```python
from build123d import *

# Parameters (mm, degrees)
BOSS_EXTRUDE1_DEPTH            = 20.32
SKETCH2_R                      = 3.175
BOSS_EXTRUDE2_DEPTH            = 69.85
F_3_5_3_5_DIAMETER_HOLE1_D     = 3.5
F_3_5_3_5_DIAMETER_HOLE1_DEPTH = 25.4
F_3_5_3_5_DIAMETER_HOLE1_TIP   = 1.051506083
F_1_16_0_0625_DIAMETER_HOLE1_D = 1.5875


with BuildPart() as part:
    # Sketch1 → Boss-Extrude1 (new body)
    with BuildSketch(Plane.XY):
        Polygon((0, 7.332348419), (-6.35, 3.666174209), (-6.35, -3.666174209), (0, -7.332348419), (6.35, -3.666174209), (6.35, 3.666174209), align=None)
    extrude(amount=BOSS_EXTRUDE1_DEPTH)

    # Sketch2 → Boss-Extrude2 (add)
    with BuildSketch(Plane.XY.offset(20.32)):
        Circle(SKETCH2_R)
    extrude(amount=BOSS_EXTRUDE2_DEPTH)

    # Ø3.5 (3.5) Diameter Hole1
    with Locations(Plane.XY.offset(90.17)):
        with Locations((0, 0)):
            Hole(F_3_5_3_5_DIAMETER_HOLE1_D / 2, depth=F_3_5_3_5_DIAMETER_HOLE1_DEPTH)
            with Locations((0, 0, -(F_3_5_3_5_DIAMETER_HOLE1_DEPTH + F_3_5_3_5_DIAMETER_HOLE1_TIP / 2))):  # 118° drill point
                Cone(0, F_3_5_3_5_DIAMETER_HOLE1_D / 2, F_3_5_3_5_DIAMETER_HOLE1_TIP, mode=Mode.SUBTRACT)

    # 1/16 (0.0625) Diameter Hole1 (through all)
    with Locations(Plane(origin=(0, 7.62, 0), x_dir=(1, 0, 0), z_dir=(0, 1, 0))):
        with Locations((0, -83.82)):
            Hole(F_1_16_0_0625_DIAMETER_HOLE1_D / 2)


solid = part.part
```
The listing builds one solid part. Answer for the finished solid, in the listing's coordinates (mm). A direction names the side the tool comes from. Give positions to 0.01 mm unless a question says otherwise; leave off trailing zeros. Write each loop counter-clockwise with the first axis right and the second up, starting at its lowest first coordinate (ties: lowest second). Pieces come first, ordered by that corner, then holes. Notation, with made-up numbers: (17, 38.5) -> (45, 38.5) arc R21 ccw to (45, 64.5) -> close; hole circle Ø1 at (-27, 18). An arc over 180 degrees is marked (long way). Write item = value, one per line. Start each with the question number.
1) Straight lines are drawn through the part: line 1 along Y through (x, z) = (0, 68.5) (3 decimals); line 2 along Z through (x, y) = (0, -2.4); line 3 along X through (y, z) = (2.3, 83.82). For each, find the intervals that lie inside material, in ascending order.
2) Which of the six approach directions +Z, -Z, +X, -X, +Y, -Y give full straight-line access (tool end or side, diameter ignored) to faces 4 (the face through (-1.617, -0.67, 77.292)), 5 (the face through (3.219, 5.474, 10.018))?
3) The part is cut by section A-A, the plane z = 83.82. Determine the outline of the cut face in (x, y) (3 decimals).
4) The part is cut by section C-C, the plane x = -4. Determine the outline of the cut face in (y, z).
5) Each of these flat-tipped pins is pushed along its axis until it touches: pin 1 (2 mm diameter, centred on x = -4.5, y = 4.5, fed in from +Z); pin 2 (5 mm diameter, centred on x = -2.5, z = 38.5, fed in from -Y) (3 decimals); pin 3 (3 mm diameter, centred on x = -4, z = 23.5, fed in from +Y). Where does it stop, or does it pass through?
6) The part is cut by section D-D, the plane y = 4.75. Determine the outline of the cut face in (x, z), and give its area (3 significant figures).
7) The part is cut by section B-B, the plane z = 50.5. Determine the outline of the cut face in (x, y) (3 decimals).
8) Determine the mould class of faces 1 (the face through (-3, -2, 20.32)), 2 (the face through (-3.131, 5.525, 10.018)), 3 (the face through (0.793, -2.379, 83.785)) for opening direction X: +X half, -X half, draft (parallel to the pull), parting line (faces both ways), or undercut.
Solutions:
q1.line_1 = -3.175 to -1.75, 1.75 to 3.175
q1.line_2 = 0 to 83.03, 84.61 to 90.17
q1.line_3 = -2.19 to -0.79, 0.79 to 2.19
q2.face_4 = +Z
q2.face_5 = +Z, -Z, +X, +Y
q3.outline = (-0.794, -3.074) -> (-0.794, -1.56) arc R1.75 cw to (-0.794, 1.56) -> (-0.794, 3.074) arc R3.175 ccw to start; (0.794, -3.074) arc R3.175 ccw to (0.794, 3.074) -> (0.794, 1.56) arc R1.75 cw to (0.794, -1.56) -> close
q4.outline = (-5.02, 0) -> (5.02, 0) -> (5.02, 20.32) -> (-5.02, 20.32) -> close
q5.pin_1 = 20.32
q5.pin_2 = -3.175
q5.pin_3 = 1.96
q6.outline = (-4.47, 0) -> (4.47, 0) -> (4.47, 20.32) -> (-4.47, 20.32) -> close
q6.area = 182 mm²
q7.outline = circle Ø6.35 at (0, 0)
q8.face_1 = draft
q8.face_2 = -X half
q8.face_3 = undercut
